from build123d import *

# Parameters (mm, degrees)
SKETCH1_R           = 14.5
BOSS_EXTRUDE1_DEPTH = 10
BOSS_EXTRUDE2_DEPTH = 20
CUT_EXTRUDE1_DEPTH  = 20
SKETCH5_W           = 10
SKETCH5_H           = 20
CUT_EXTRUDE2_DEPTH  = 20
SKETCH6_R           = 2.85
BOSS_EXTRUDE3_DEPTH = 1
SCALE1_SCALE        = 0.5
SKETCH7_R           = 4.75
BOSS_EXTRUDE4_DEPTH = 35


with BuildPart() as part:
    # Sketch1 → Boss-Extrude1 (new body)
    with BuildSketch(Plane(origin=(0, 0, 0), x_dir=(1, 0, 0), z_dir=(0, 1, 0))):
        with Locations(Location((0, 0, 0), (0, 0, 270))):
            Circle(SKETCH1_R)
    extrude(amount=BOSS_EXTRUDE1_DEPTH)

    # Sketch2 → Boss-Extrude2 (add)
    with BuildSketch(Plane(origin=(0, 10, 0), x_dir=(1, 0, 0), z_dir=(0, 1, 0))):
        Polygon((-10, 0), (-10, 10), (10, 10), (10, -10), (-10, -10), align=None)
    extrude(amount=BOSS_EXTRUDE2_DEPTH)

    # Sketch3 → Cut-Extrude1 (cut)
    with BuildSketch(Plane.ZY.offset(10)):
        with BuildLine():
            Line((-6.5, 23), (-6.5, 10))
            Line((-6.5, 10), (-10, 10))
            Line((-10, 10), (-10, 30))
            Line((-10, 30), (10, 30))
            Line((10, 30), (10, 10))
            Line((10, 10), (6.5, 10))
            Line((6.5, 10), (6.5, 23))
            ThreePointArc((6.5, 23), (0, 29.5), (-6.5, 23))
        make_face()
    extrude(amount=-CUT_EXTRUDE1_DEPTH, mode=Mode.SUBTRACT)

    # Sketch5 → Cut-Extrude2 (cut)
    with BuildSketch(Plane.XY.offset(6.5)):
        with Locations((0, 20)):
            Rectangle(SKETCH5_W, SKETCH5_H)
    extrude(amount=-CUT_EXTRUDE2_DEPTH, mode=Mode.SUBTRACT)

    # Sketch6 → Boss-Extrude3 (add)
    with BuildSketch(Plane(origin=(-5, 0, 0), x_dir=(0, 0, -1), z_dir=(1, 0, 0))):
        with Locations(Location((0, 23, 0), (0, 0, 270))):
            Circle(SKETCH6_R)
    boss_extrude3 = extrude(amount=BOSS_EXTRUDE3_DEPTH)

    # Mirror1: Boss-Extrude3 across plane
    add(boss_extrude3.mirror(Plane(origin=(0, 0, 0), x_dir=(0, 0, 1), z_dir=(1, 0, 0))))


with BuildPart() as part_1:
    # Scale1: scaled about (0, 0, 0)
    add(part.part.scale(SCALE1_SCALE))

    # Sketch7 → Boss-Extrude4 (add)
    with BuildSketch(Plane.XZ):
        with Locations(Location((0, 0, 0), (0, 0, 270))):
            Circle(SKETCH7_R)
    extrude(amount=BOSS_EXTRUDE4_DEPTH)

    # Sketch8 → Revolve1 (revolve)
    with BuildSketch(Plane.XY, mode=Mode.PRIVATE) as revolve1_sk:
        Polygon((0, -35), (4.75, -35), (0, -46.4), align=None)
    revolve(revolve1_sk.sketch.rotate(Axis((0, -35, 0), (0, -1, 0)), 90), axis=Axis((0, -35, 0), (0, -1, 0)))


solid = part_1.part
The listing builds one solid part. Answer for the finished solid, in the listing's coordinates (mm). A direction names the side the tool comes from. Coordinates: 2 decimals unless noted, no trailing zeros. Loops run counter-clockwise (first coordinate to the right, second up) from the corner with the lowest first, then second, coordinate; pieces in that order, holes last. Notation, with made-up numbers: (12, 14.25) -> (30, 14.25) arc R23 ccw to (30, 27.25) -> close; hole circle Ø2 at (38.25, 21). An arc over 180 degrees is marked (long way). Answer in a Markdown table with one row per item. Add a question column.
1. For faces 1 (the flat face through (-4, 8, -3.25)), 2 (the flat face through (5, 10, 0)), 3 (the flat face through (-2, 12, 0)), 4 (the flat face through (4, 8, 3.25)), 5 (the cylindrical face through (2.25, 11.81, 1.39)), determine the directions among +Z, -Z, +X, -X, +Y, -Y from which every point of the face is accessible in a straight line to the end or side of a thin tool.
2. The part is cut by section B-B, the plane z = -5.75. Write down the section's boundary in (x, y), then the cut area to 3 significant figures.
3. Flat-ended cylindrical pins translate along their axes: P1, Ø3, axis at y = 4, z = 2.5, coming from the -X side; P2, Ø7, axis at y = 10, z = 0.5, coming from the +X side; P3, Ø2, axis at x = -3, y = 7.5, coming from the +Z side. Find the tip coordinate at first contact, or state that the pin passes through.
4. The part is cut by section C-C, the plane y = -40. Write down the section's boundary in (x, z), then the cut area to 3 significant figures.
5. Determine the mould class of faces 6 (the cylindrical face through (-2.25, 11.81, 1.39)), 7 (the cylindrical face through (-3.77, 14.75, 0.07)), 8 (the flat face through (-4, 8, 3.25)), 9 (the conical face through (-0.54, -42.05, 1.73)) for opening direction Y: +Y half, -Y half, draft (parallel to the pull), parting line (faces both ways), or undercut.
6. The part is cut by section A-A, the plane y = -25.5. Write down the section's boundary in (x, z).
7. Consider line 1 (Y direction, x = -0.25, z = -6.5); line 2 (X direction, y = 9, z = 0); line 3 (Z direction, x = 0.25, y = -18). Determine where each line is inside the solid, lowest interval first. Write a range as [from, to].
Answer below:
| question | item | result |
|---|---|---|
| 1 | face 1 | -Z, +X, -X, +Y |
| 1 | face 2 | +Z, -Z, +X, +Y |
| 1 | face 3 | +Z, -Z, +Y |
| 1 | face 4 | +Z, +X, -X, +Y |
| 1 | face 5 | none |
| 2 | outline | (-4.42, 0) -> (4.42, 0) -> (4.42, 5) -> (-4.42, 5) -> close |
| 2 | area | 44.2 mm2 |
| 3 | P1 | x = -7.18 |
| 3 | P2 | x = 5 |
| 3 | P3 | z = 3.25 |
| 4 | outline | circle Ø5.33 at (0, 0) |
| 4 | area | 22.3 mm2 |
| 5 | face 6 | undercut |
| 5 | face 7 | +Y half |
| 5 | face 8 | draft |
| 5 | face 9 | -Y half |
| 6 | outline | circle Ø9.5 at (0, 0) |
| 7 | line 1 | [0, 5] |
| 7 | line 2 | [-5, -2.5], [2.5, 5] |
| 7 | line 3 | [-4.74, 4.74] |
